Autodesk Inventor part; units mm, degrees
ref_plane "YZ Plane" through (0, 0, 0) normal (1, 0, 0) x (0, 1, 0)
ref_plane "XZ Plane" through (0, 0, 0) normal (0, 1, 0) x (-1, 0, 0)
ref_plane "XY Plane" through (0, 0, 0) normal (0, 0, 1) x (1, 0, 0)
sketch "스케치1" plane through (0, 0, 0) normal (0, 0, 1) x (1, 0, 0)
  circle A0 centre (0, 0) radius 20
  dimension "d0" = 40
extrude "돌출1" add sketch "스케치1" along normal blind 30
sketch "스케치2" plane through (0, 0, 30) normal (0, 0, 1) x (1, 0, 0)
  circle A0 centre (0, 0) radius 15
  dimension "d3" = 30
extrude "돌출2" add sketch "스케치2" along normal blind 40
sketch "스케치3" plane through (0, 0, 0) normal (0, 0, -1) x (-1, 0, 0)
  circle A0 centre (0, 0) radius 12.5
  dimension "d6" = 25
extrude "돌출3" cut sketch "스케치3" against normal blind 30
sketch "스케치4" plane through (0, 0, 30) normal (0, 0, -1) x (-1, 0, 0)
  circle A0 centre (0, 0) radius 7.5
  dimension "d9" = 15
extrude "돌출4" cut sketch "스케치4" against normal blind 20
sketch "스케치5" plane through (0, 0, 50) normal (0, 0, -1) x (-1, 0, 0)
  circle A0 centre (0, 0) radius 10
  dimension "d12" = 20
extrude "돌출5" cut sketch "스케치5" against normal up to next
properties part number "기본 투상 연습2"
Here's how the part is built. I have some questions about the finished solid (model axes, mm). A direction names the side the tool comes from. Coordinates: 2 decimals unless noted, no trailing zeros. Loops run counter-clockwise (first coordinate to the right, second up) from the corner with the lowest first, then second, coordinate; pieces in that order, holes last. Notation, with made-up numbers: (59, 48.25) - (75, 48.25) arc R26 cw to (75, 67.25) - close; hole circle Ø7 at (56, 79.25). An arc over 180 degrees is marked (long way). Answer as CSV lines item,"result".
Q1. For pin 1 (3 mm diameter, centred on x = 6, y = -6, fed in from -Z); pin 2 (3 mm diameter, centred on y = -4.5, z = 60, fed in from +X); pin 3 (3 mm diameter, centred on x = 7.5, z = 43, fed in from +Y), each with a flat end and sliding along its axis, tell me the tip position at first contact or that it passes through.
Response:
pin 1,"z = 30"
pin 2,"x = 14.7"
pin 3,"y = 13.75"
Q2. We'd pull the mould along X, two halves only. Please class faces 1 (the face through (-14.985, -0.66, 49.72)), 2 (the face through (7.493, 0.33, 39.86)), 3 (the face through (9, 9, 0)), 4 (the face through (-4, 7, 50)): pulls with the +X half, pulls with the -X half, needs draft (parallel to the pull), parting line crosses it, or undercut.
Response:
face 1,"parting line crosses it"
face 2,"undercut"
face 3,"needs draft"
face 4,"undercut"
Q3. If we section it at A-A, the plane y = 0: Write out the boundary of the cut face in (x, z).
Response:
outline,"(-20, 0) - (-12.5, 0) - (-12.5, 30) - (-7.5, 30) - (-7.5, 50) - (-10, 50) - (-10, 70) - (-15, 70) - (-15, 30) - (-20, 30) - close; (7.5, 30) - (12.5, 30) - (12.5, 0) - (20, 0) - (20, 30) - (15, 30) - (15, 70) - (10, 70) - (10, 50) - (7.5, 50) - close"
Q4. If we section it at D-D, the plane x = -13.5: Write out the boundary of the cut face in (y, z), and give its area (3 significant figures).
Response:
outline,"(-14.76, 0) - (14.76, 0) - (14.76, 30) - (6.54, 30) - (6.54, 70) - (-6.54, 70) - (-6.54, 30) - (-14.76, 30) - close"
area,"1,410 mm2"
Q5. If we section it at C-C, the plane z = 40.5: Write out the boundary of the cut face in (x, y), and give its area (3 significant figures).
Response:
outline,"circle Ø30 at (0, 0); hole circle Ø15 at (0, 0)"
area,"530 mm2"
Q6. For faces 5 (the face through (-4.336, 19.524, 14.79)), 6 (the face through (0, -8, 30)), 7 (the face through (3, 15, 30)), which set-ups out of +Z, -Z, +X, -X, +Y, -Y let a thin tool reach every point of the face, with its end or its side?
Response:
face 5,"+Z, -Z"
face 6,"-Z"
face 7,"+Z"
Q7. If I drill on L1, parallel to Y at x = 0, z = 38; L2, parallel to Y at x = 0, z = 56.75; L3, parallel to Z at x = 15.5, y = 0.5, over which ranges is the centre line in solid material (lowest first)? Write a range as [from, to].
Response:
L1,"[-15, -7.5], [7.5, 15]"
L2,"[-15, -10], [10, 15]"
L3,"[0, 30]"
